from build123d import *

# Parameters (mm, degrees)
SKETCH1_R           = 63.5
SKETCH1_R_2         = 19.05
BOSS_EXTRUDE1_DEPTH = 25.4
CUT_EXTRUDE1_DEPTH  = 6.35
CUT_EXTRUDE2_START  = -6.35
CUT_EXTRUDE2_DEPTH  = 6.35


with BuildPart() as part:
    # Sketch1 → Boss-Extrude1 (new, symmetric)
    with BuildSketch(Plane.XY):
        Circle(SKETCH1_R)
        Circle(SKETCH1_R_2, mode=Mode.SUBTRACT)
    extrude(amount=BOSS_EXTRUDE1_DEPTH, both=True)

    # Sketch3 → Cut-Extrude1 (cut)
    with BuildSketch(Plane.XY.offset(25.4)):
        with BuildLine():
            Line((36.77386566, 22.631730036), (47.770554295, 33.628418671))
            ThreePointArc((47.770554295, 33.628418671), (53.973042289, 22.356366119), (57.557765766, 10))
            Line((57.557765766, 10), (42.006099557, 10))
            ThreePointArc((42.006099557, 10), (39.893118214, 16.52427061), (36.77386566, 22.631730036))
        make_face()
        with BuildLine():
            Line((47.770554295, -33.628418671), (36.77386566, -22.631730036))
            ThreePointArc((36.77386566, -22.631730036), (39.893118214, -16.52427061), (42.006099557, -10))
            Line((42.006099557, -10), (57.557765766, -10))
            ThreePointArc((57.557765766, -10), (53.973042289, -22.356366119), (47.770554295, -33.628418671))
        make_face()
        with BuildLine():
            Line((10, -57.557765766), (10, -42.006099557))
            ThreePointArc((10, -42.006099557), (16.52427061, -39.893118214), (22.631730036, -36.77386566))
            Line((22.631730036, -36.77386566), (33.628418671, -47.770554295))
            ThreePointArc((33.628418671, -47.770554295), (22.356366119, -53.973042289), (10, -57.557765766))
        make_face()
        with BuildLine():
            Line((-33.628418671, -47.770554295), (-22.631730036, -36.77386566))
            ThreePointArc((-22.631730036, -36.77386566), (-16.52427061, -39.893118214), (-10, -42.006099557))
            Line((-10, -42.006099557), (-10, -57.557765766))
            ThreePointArc((-10, -57.557765766), (-22.356366119, -53.973042289), (-33.628418671, -47.770554295))
        make_face()
        with BuildLine():
            Line((-42.006099557, 10), (-57.557765766, 10))
            ThreePointArc((-57.557765766, 10), (-53.973042289, 22.356366119), (-47.770554295, 33.628418671))
            Line((-47.770554295, 33.628418671), (-36.77386566, 22.631730036))
            ThreePointArc((-36.77386566, 22.631730036), (-39.893118214, 16.52427061), (-42.006099557, 10))
        make_face()
        with BuildLine():
            Line((22.631730036, 36.77386566), (33.628418671, 47.770554295))
            ThreePointArc((33.628418671, 47.770554295), (22.356366119, 53.973042289), (10, 57.557765766))
            Line((10, 57.557765766), (10, 42.006099557))
            ThreePointArc((10, 42.006099557), (16.52427061, 39.893118214), (22.631730036, 36.77386566))
        make_face()
        with BuildLine():
            Line((-47.770554295, -33.628418671), (-36.77386566, -22.631730036))
            ThreePointArc((-36.77386566, -22.631730036), (-39.893118214, -16.52427061), (-42.006099557, -10))
            Line((-42.006099557, -10), (-57.557765766, -10))
            ThreePointArc((-57.557765766, -10), (-53.973042289, -22.356366119), (-47.770554295, -33.628418671))
        make_face()
        with BuildLine():
            Line((-22.631730036, 36.77386566), (-33.628418671, 47.770554295))
            ThreePointArc((-33.628418671, 47.770554295), (-22.356366119, 53.973042289), (-10, 57.557765766))
            Line((-10, 57.557765766), (-10, 42.006099557))
            ThreePointArc((-10, 42.006099557), (-16.52427061, 39.893118214), (-22.631730036, 36.77386566))
        make_face()
    extrude(amount=-CUT_EXTRUDE1_DEPTH, mode=Mode.SUBTRACT)

    # Sketch4 → Cut-Extrude2 (cut)
    with BuildSketch(Plane(origin=(0, 0, -25.4), x_dir=(-1, 0, 0), z_dir=(0, 0, -1)).offset(CUT_EXTRUDE2_START)):
        with BuildLine():
            Line((-36.77386566, -22.631730036), (-47.770554295, -33.628418671))
            ThreePointArc((-47.770554295, -33.628418671), (-53.973042289, -22.356366119), (-57.557765766, -10))
            Line((-57.557765766, -10), (-42.006099557, -10))
            ThreePointArc((-42.006099557, -10), (-39.893118214, -16.52427061), (-36.77386566, -22.631730036))
        make_face()
        with BuildLine():
            Line((-10, -42.006099557), (-10, -57.557765766))
            ThreePointArc((-10, -57.557765766), (-22.356366119, -53.973042289), (-33.628418671, -47.770554295))
            Line((-33.628418671, -47.770554295), (-22.631730036, -36.77386566))
            ThreePointArc((-22.631730036, -36.77386566), (-16.52427061, -39.893118214), (-10, -42.006099557))
        make_face()
        with BuildLine():
            Line((22.631730036, -36.77386566), (33.628418671, -47.770554295))
            ThreePointArc((33.628418671, -47.770554295), (22.356366119, -53.973042289), (10, -57.557765766))
            Line((10, -57.557765766), (10, -42.006099557))
            ThreePointArc((10, -42.006099557), (16.52427061, -39.893118214), (22.631730036, -36.77386566))
        make_face()
        with BuildLine():
            Line((42.006099557, -10), (57.557765766, -10))
            ThreePointArc((57.557765766, -10), (53.973042289, -22.356366119), (47.770554295, -33.628418671))
            Line((47.770554295, -33.628418671), (36.77386566, -22.631730036))
            ThreePointArc((36.77386566, -22.631730036), (39.893118214, -16.52427061), (42.006099557, -10))
        make_face()
        with BuildLine():
            Line((36.77386566, 22.631730036), (47.770554295, 33.628418671))
            ThreePointArc((47.770554295, 33.628418671), (53.973042289, 22.356366119), (57.557765766, 10))
            Line((57.557765766, 10), (42.006099557, 10))
            ThreePointArc((42.006099557, 10), (39.893118214, 16.52427061), (36.77386566, 22.631730036))
        make_face()
        with BuildLine():
            Line((10, 42.006099557), (10, 57.557765766))
            ThreePointArc((10, 57.557765766), (22.356366119, 53.973042289), (33.628418671, 47.770554295))
            Line((33.628418671, 47.770554295), (22.631730036, 36.77386566))
            ThreePointArc((22.631730036, 36.77386566), (16.52427061, 39.893118214), (10, 42.006099557))
        make_face()
        with BuildLine():
            Line((-22.631730036, 36.77386566), (-33.628418671, 47.770554295))
            ThreePointArc((-33.628418671, 47.770554295), (-22.356366119, 53.973042289), (-10, 57.557765766))
            Line((-10, 57.557765766), (-10, 42.006099557))
            ThreePointArc((-10, 42.006099557), (-16.52427061, 39.893118214), (-22.631730036, 36.77386566))
        make_face()
        with BuildLine():
            Line((-42.006099557, 10), (-57.557765766, 10))
            ThreePointArc((-57.557765766, 10), (-53.973042289, 22.356366119), (-47.770554295, 33.628418671))
            Line((-47.770554295, 33.628418671), (-36.77386566, 22.631730036))
            ThreePointArc((-36.77386566, 22.631730036), (-39.893118214, 16.52427061), (-42.006099557, 10))
        make_face()
    extrude(amount=CUT_EXTRUDE2_DEPTH, mode=Mode.SUBTRACT)


solid = part.part
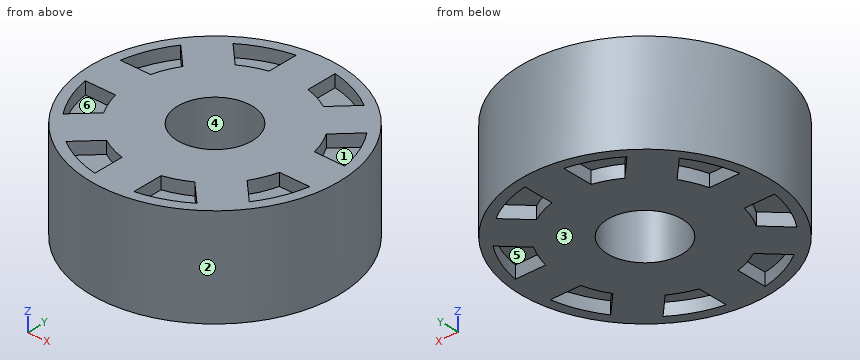
Geometry: final body of the model. Coordinates: model frame, mm. Face numbers are marked on the shaded views. A direction names the side the tool comes from. Give positions to 0.01 mm unless a question says otherwise; leave off trailing zeros. Loops run counter-clockwise (first coordinate to the right, second up) from the corner with the lowest first, then second, coordinate; pieces in that order, holes last. Notation, with made-up numbers: (26.5, -17.5) -> (32.5, -17.5) arc R23 ccw to (32.5, -6.5) -> close; hole circle Ø3 at (18, -25.5). An arc over 180 degrees is marked (long way). Put each result on its own line as item: value.
1. Set-up query: the marked faces 4, 5 and 6. Return all of +Z, -Z, +X, -X, +Y, -Y with unobstructed straight access to the full face (end or side cutting, diameter ignored); none if empty.
Taken from the geometry:
face 4: +Z, -Z
face 5: -Z
face 6: +Z
2. Pull-direction query (X, two-part tool) for the marked faces 1, 2 and 3; classes: released by +X, released by -X, zero draft, split by the parting line, or undercut.
Taken from the geometry:
face 1: undercut
face 2: split by the parting line
face 3: zero draft
3. Ray query, line 1 along X through (y, z) = (23, 20.5); line 2 along Y through (x, z) = (0, 11); line 3 along X through (y, z) = (28, -22). Return the intervals inside material, ascending. Write a range as [from, to].
Taken from the geometry:
line 1: x = [-59.19, -53.7], [-37.14, 37.14], [53.7, 59.19]
line 2: y = [-63.5, -19.05], [19.05, 63.5]
line 3: x = [-56.99, -51.27], [-42.14, 42.14], [51.27, 56.99]
4. Cut plane A-A (y = 0). Return the cut outline in (x, z), plus the area to 3 significant figures.
Taken from the geometry:
outline: (-63.5, -25.4) -> (-19.05, -25.4) -> (-19.05, 25.4) -> (-63.5, 25.4) -> close; (19.05, -25.4) -> (63.5, -25.4) -> (63.5, 25.4) -> (19.05, 25.4) -> close
area: 4,520 mm2
5. Pin query (flat end, axial travel): P1, Ø4, axis at y = -40, z = -13.5, coming from the -X side; P2, Ø7, axis at x = -50, z = -23, coming from the +Y side; P3, Ø10, axis at x = -42, z = -17, coming from the -Y side. Return the tip coordinate at first contact, or that it passes through.
Taken from the geometry:
P1: stops at x = -50.87
P2: stops at y = 43.24
P3: stops at y = -51.61
6. Cut plane C-C (x = -32). Return the cut outline in (y, z).
Taken from the geometry:
outline: (-54.85, -25.4) -> (-48.88, -25.4) -> (-48.88, -19.05) -> (-46.14, -19.05) -> (-46.14, -25.4) -> (46.14, -25.4) -> (46.14, -19.05) -> (48.88, -19.05) -> (48.88, -25.4) -> (54.85, -25.4) -> (54.85, 25.4) -> (48.88, 25.4) -> (48.88, 19.05) -> (46.14, 19.05) -> (46.14, 25.4) -> (-46.14, 25.4) -> (-46.14, 19.05) -> (-48.88, 19.05) -> (-48.88, 25.4) -> (-54.85, 25.4) -> close
7. Cut plane D-D (y = -46). Return the cut outline in (x, z) (3 decimals), plus the area to 3 significant figures.
Taken from the geometry:
outline: (-43.775, -25.4) -> (-31.858, -25.4) -> (-31.858, -19.05) -> (-10, -19.05) -> (-10, -25.4) -> (10, -25.4) -> (10, -19.05) -> (31.858, -19.05) -> (31.858, -25.4) -> (43.775, -25.4) -> (43.775, 25.4) -> (31.858, 25.4) -> (31.858, 19.05) -> (10, 19.05) -> (10, 25.4) -> (-10, 25.4) -> (-10, 19.05) -> (-31.858, 19.05) -> (-31.858, 25.4) -> (-43.775, 25.4) -> close
area: 3,890 mm2
